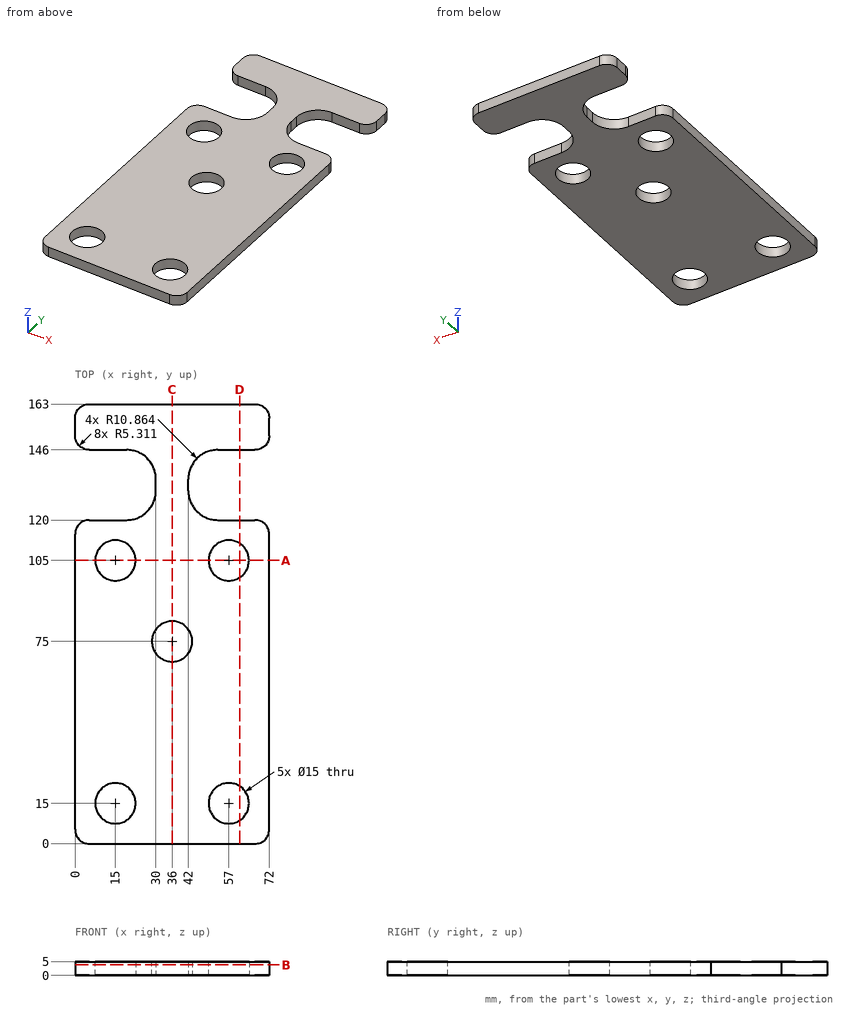
Study the drawing (mm; zero at the part's minimum x, y, z) and answer. Give positions to 0.01 mm unless a question says otherwise; leave off trailing zeros. Write each loop counter-clockwise with the first axis right and the second up, starting at its lowest first coordinate (ties: lowest second). Pieces come first, ordered by that corner, then holes. Notation, with made-up numbers: (-25, -34.5) -> (22, -34.5) arc R5 cw to (22, -26.5) -> close; hole circle Ø3 at (62.25, 6.5). An arc over 180 degrees is marked (long way). Write item = value, one per line. Start each with the question number.
1) Each of these flat-tipped pins is pushed along its axis until it touches: pin 1 (1.3 mm diameter, centred on y = 132.5, z = 3, fed in from -X); pin 2 (12 mm diameter, centred on x = 57, y = 15, fed in from +Z). Where does it stop, or does it pass through?
2) The part is cut by section D-D, the plane x = 61. Determine the outline of the cut face in (y, z).
3) The part is cut by section A-A, the plane y = 105. Determine the outline of the cut face in (x, z).
4) The part is cut by section C-C, the plane x = 36. Determine the outline of the cut face in (y, z).
5) Straight lines are drawn through the part: line 1 along Y through (x, z) = (57, 1.1); line 2 along Y through (x, z) = (36, 1.15); line 3 along Y through (x, z) = (21, 3.5). For each, find the intervals that lie inside material, in ascending order.
6) The part is cut by section B-B, the plane z = 3.85. Count the separate pieces of the cut face and the enclosed holes in it.
Solutions:
q1.pin_1 = 30
q1.pin_2 = through
q2.outline = (0, 0) -> (8.66, 0) -> (8.66, 5) -> (0, 5) -> close; (21.34, 0) -> (98.66, 0) -> (98.66, 5) -> (21.34, 5) -> close; (111.34, 0) -> (120, 0) -> (120, 5) -> (111.34, 5) -> close; (146, 0) -> (163, 0) -> (163, 5) -> (146, 5) -> close
q3.outline = (0, 0) -> (7.5, 0) -> (7.5, 5) -> (0, 5) -> close; (22.5, 0) -> (49.5, 0) -> (49.5, 5) -> (22.5, 5) -> close; (64.5, 0) -> (72, 0) -> (72, 5) -> (64.5, 5) -> close
q4.outline = (0, 0) -> (67.5, 0) -> (67.5, 5) -> (0, 5) -> close; (82.5, 0) -> (163, 0) -> (163, 5) -> (82.5, 5) -> close
q5.line_1 = 0 to 7.5, 22.5 to 97.5, 112.5 to 120, 146 to 163
q5.line_2 = 0 to 67.5, 82.5 to 163
q5.line_3 = 0 to 10.5, 19.5 to 100.5, 109.5 to 120.16, 145.84 to 163
q6.separate_pieces = 1
q6.enclosed_holes = 5
